```python
from build123d import *

# Parameters (mm, degrees)
SKETCH1_R           = 0.9525
BOSS_EXTRUDE1_DEPTH = 9.525
SKETCH2_R           = 1.5875
BOSS_EXTRUDE2_DEPTH = 1.905


with BuildPart() as part:
    # Sketch1 → Boss-Extrude1 (new body)
    with BuildSketch(Plane(origin=(0, 0, 0), x_dir=(1, 0, 0), z_dir=(0, 1, 0))):
        Circle(SKETCH1_R)
    boss_extrude1 = extrude(amount=BOSS_EXTRUDE1_DEPTH)

    # Sketch2 → Boss-Extrude2 (add)
    with BuildSketch(Plane(origin=(0, 9.525, 0), x_dir=(1, 0, 0), z_dir=(0, 1, 0))):
        Circle(SKETCH2_R)
    boss_extrude2 = extrude(amount=BOSS_EXTRUDE2_DEPTH)

    # Mirror1: Boss-Extrude1, Boss-Extrude2 across plane
    add(boss_extrude1.mirror(Plane.ZX))
    add(boss_extrude2.mirror(Plane.ZX))


solid = part.part
```
The listing builds one solid part. Answer for the finished solid, in the listing's coordinates (mm). A direction names the side the tool comes from. Give positions to 0.01 mm unless a question says otherwise; leave off trailing zeros. Loops run counter-clockwise (first coordinate to the right, second up) from the corner with the lowest first, then second, coordinate; pieces in that order, holes last. Notation, with made-up numbers: (-25.5, -11) - (-6.5, -11) arc R9 cw to (-6.5, -3) - close; hole circle Ø1 at (74.5, 44). An arc over 180 degrees is marked (long way). Answer as CSV lines item,"result". Start each with the question number.
Item 1: A cutting plane is placed at B-B on z = 0. Determine the outline of the cut face in (x, y) (1 decimal), then the cut area to 3 significant figures.
Item 2: A cutting plane is placed at D-D on y = 2.5. Determine the outline of the cut face in (x, z) (1 decimal), then the cut area to 3 significant figures.
Item 3: Find the intervals of material crossed by line 1 (Y direction, x = -0.9, z = 1.15) (3 decimals); line 2 (X direction, y = 10.75, z = -0.4); line 3 (Z direction, x = -0.3, y = -4.25), in increasing order. Write a range as from..to.
Item 4: A cutting plane is placed at C-C on x = 0. Determine the outline of the cut face in (y, z) (1 decimal), then the cut area to 3 significant figures.
Item 5: This flat-tipped pin is pushed along its axis until it touches: pin 1 (1.5 mm diameter, centred on y = -8.5, z = -0.5, fed in from -X). Where does it stop, or does it pass through?
Item 6: A cutting plane is placed at A-A on x = 1.2. Determine the outline of the cut face in (y, z) (3 decimals), then the cut area to 3 significant figures.
Item 7: The mould has two halves that part along Y. Classify faces 1 (the face through (0, -11.43, 0)), 2 (the face through (1, 9.525, 1)), 3 (the face through (0, 11.43, 0)), 4 (the face through (-0.34, -10.46, 1.55)): +Y half, -Y half, draft (parallel to the pull), parting line (faces both ways), or undercut.
Item 8: For faces 5 (the face through (-0.34, 10.46, 1.55)), 6 (the face through (-0.21, 0.13, 0.93)), determine the directions among +Z, -Z, +X, -X, +Y, -Y from which every point of the face is accessible in a straight line to the end or side of a thin tool.
Found:
1,outline,"(-1.6, -11.4) - (1.6, -11.4) - (1.6, -9.5) - (1, -9.5) - (1, 9.5) - (1.6, 9.5) - (1.6, 11.4) - (-1.6, 11.4) - (-1.6, 9.5) - (-1, 9.5) - (-1, -9.5) - (-1.6, -9.5) - close"
1,area,"48.4 mm^2"
2,outline,"circle Ø1.9 at (0, 0)"
2,area,"2.85 mm^2"
3,line 1,"y = -11.43..-9.525, 9.525..11.43"
3,line 2,"x = -1.54..1.54"
3,line 3,"z = -0.9..0.9"
4,outline,"(-11.4, -1.6) - (-9.5, -1.6) - (-9.5, -1) - (9.5, -1) - (9.5, -1.6) - (11.4, -1.6) - (11.4, 1.6) - (9.5, 1.6) - (9.5, 1) - (-9.5, 1) - (-9.5, 1.6) - (-11.4, 1.6) - close"
4,area,"48.4 mm^2"
5,pin 1,"stops at x = -0.95"
6,outline,"(-11.43, -1.039) - (-9.525, -1.039) - (-9.525, 1.039) - (-11.43, 1.039) - close; (9.525, -1.039) - (11.43, -1.039) - (11.43, 1.039) - (9.525, 1.039) - close"
6,area,"7.92 mm^2"
7,face 1,"-Y half"
7,face 2,"undercut"
7,face 3,"+Y half"
7,face 4,"draft"
8,face 5,"+Y, -Y"
8,face 6,"none"
